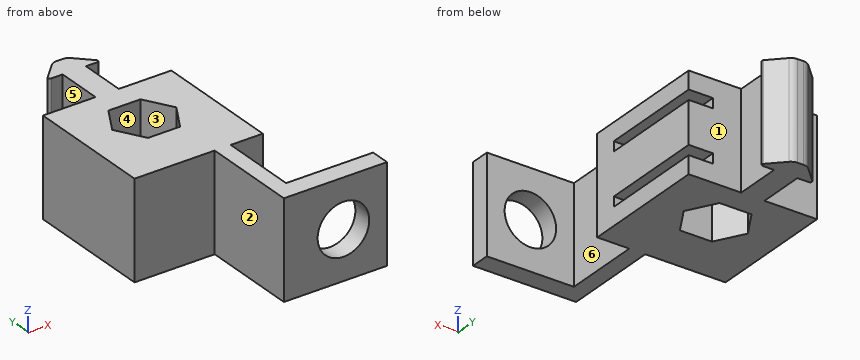
```python
from build123d import *

# Parameters (mm, degrees)
BOSS_EXTRUDE1_DEPTH = 12.7
SKETCH8_W           = 2.54
SKETCH8_H           = 27.5
CUT_EXTRUDE1_DEPTH  = 6.35
SKETCH3_W           = 4.197769469
SKETCH3_H           = 25.4
BOSS_EXTRUDE2_DEPTH = 25.4
SKETCH4_W           = 22.800422122
SKETCH4_H           = 25.4
SKETCH4_R           = 6.75
BOSS_EXTRUDE3_DEPTH = 5.08


with BuildPart() as part:
    # Sketch1 → Boss-Extrude1 (new body, symmetric)
    with BuildSketch(Plane.XY):
        with BuildLine():
            Line((-16.79575, 13.62075), (-16.79575, -19.97075))
            Line((-16.79575, -19.97075), (16.79575, -19.97075))
            Line((16.79575, -19.97075), (16.79575, 13.62075))
            Line((16.79575, 13.62075), (3.048, 13.62075))
            Line((3.048, 13.62075), (3.048, 25.68575))
            Line((3.048, 25.68575), (6.01257951, 25.68575))
            ThreePointArc((6.01257951, 25.68575), (6.481910313, 25.999346816), (6.371789755, 26.552960245))
            Line((6.371789755, 26.552960245), (2.532108776, 30.392641224))
            ThreePointArc((2.532108776, 30.392641224), (1.70807347, 30.943244013), (0.736057552, 31.13659))
            Line((0.736057552, 31.13659), (-0.736057552, 31.13659))
            ThreePointArc((-0.736057552, 31.13659), (-1.70807347, 30.943244013), (-2.532108776, 30.392641224))
            Line((-2.532108776, 30.392641224), (-6.371789755, 26.552960245))
            ThreePointArc((-6.371789755, 26.552960245), (-6.481910313, 25.999346816), (-6.01257951, 25.68575))
            Line((-6.01257951, 25.68575), (-3.048, 25.68575))
            Line((-3.048, 25.68575), (-3.048, 13.62075))
            Line((-3.048, 13.62075), (-16.79575, 13.62075))
        make_face()
        Polygon((-4.19776947, 7.27075), (-8.395538939, 0), (-4.19776947, -7.27075), (4.19776947, -7.27075), (8.395538939, 0), (4.19776947, 7.27075), align=None, mode=Mode.SUBTRACT)
    extrude(amount=BOSS_EXTRUDE1_DEPTH, both=True)

    # Sketch8 → Cut-Extrude1 (cut)
    with BuildSketch(Plane(origin=(16.79575, 0, 0), x_dir=(0, 0, -1), z_dir=(1, 0, 0))):
        with Locations((-6.77, -0.12925)):
            Rectangle(SKETCH8_W, SKETCH8_H)
        with Locations((6.77, -0.12925)):
            Rectangle(SKETCH8_W, SKETCH8_H)
    extrude(amount=-CUT_EXTRUDE1_DEPTH, mode=Mode.SUBTRACT)

    # Sketch3 → Boss-Extrude2 (add)
    with BuildSketch(Plane.XZ.offset(19.97075)):
        with Locations((6.296654204, 0)):
            Rectangle(SKETCH3_W, SKETCH3_H)
    extrude(amount=BOSS_EXTRUDE2_DEPTH)

    # Sketch4 → Boss-Extrude3 (add)
    with BuildSketch(Plane.XZ.offset(45.37075)):
        with Locations((19.79575, 0)):
            Rectangle(SKETCH4_W, SKETCH4_H)
        with Locations((19.79575, 0)):
            Circle(SKETCH4_R, mode=Mode.SUBTRACT)
    extrude(amount=-BOSS_EXTRUDE3_DEPTH)


solid = part.part
```
For this review, take the finished solid that the model builds, in its own axes (mm). Face numbers are marked on the shaded views. A direction names the side the tool comes from. Coordinates: 2 decimals unless noted, no trailing zeros. Write each loop counter-clockwise with the first axis right and the second up, starting at its lowest first coordinate (ties: lowest second). Pieces come first, ordered by that corner, then holes.
(1) For pin 1 Ø6 at (y, z) = (-34.5, 7) entering from -X; pin 2 Ø1.5 at (x, z) = (5.5, -6) entering from +Y; pin 3 Ø0.9 at (x, z) = (-5, -6) entering from -Y, all flat-tipped, find the tip position at first contact; note any pin that passes through.
(2) Add section C-C on y = 8.5. Give the boundary of the cut face in (x, z), then the cut area to 3 significant figures.
(3) Tool access review of the marked faces 4, 5 and 6: name each direction out of +Z, -Z, +X, -X, +Y, -Y from which nothing blocks a thin tool from reaching the whole face with its end or side.
(4) Add section A-A on z = 0. Count the separate pieces of the cut face and the enclosed holes in it, then the cut area to 3 significant figures.
(5) Add section B-B on z = -9.5. Give the boundary of the cut face in (x, y).
(6) The part is to be moulded in two halves that separate along X. For the marked faces 1, 2 and 3, say which applies: +X half, -X half, draft (parallel to the pull), parting line (faces both ways), or undercut.
(7) Wall thickness on probe 1 along Y at (x, z) = (12, 7.5); probe 2 along Y at (x, z) = (11, -3); probe 3 along X at (y, z) = (-5, 4.75): over which ranges is each line inside the solid? List them lowest first.
Answer sheet:
1. pin 1: stops at x = 4.2
1. pin 2: stops at y = 28.17
1. pin 3: stops at y = -19.97
2. outline: (-16.8, -12.7) - (16.8, -12.7) - (16.8, -8.04) - (10.45, -8.04) - (10.45, -5.5) - (16.8, -5.5) - (16.8, 5.5) - (10.45, 5.5) - (10.45, 8.04) - (16.8, 8.04) - (16.8, 12.7) - (-16.8, 12.7) - close
2. area: 821 mm2
3. face 4: +Z, -Z
3. face 5: +Z, -Z, -X
3. face 6: +Z, -Z, +X
4. separate pieces: 2
4. enclosed holes: 1
4. area: 1,220 mm2
5. outline: (-16.8, -19.97) - (4.2, -19.97) - (4.2, -45.37) - (31.2, -45.37) - (31.2, -40.29) - (8.4, -40.29) - (8.4, -19.97) - (16.8, -19.97) - (16.8, 13.62) - (3.05, 13.62) - (3.05, 25.69) - (6.01, 25.69) arc R0.51 ccw to (6.37, 26.55) - (2.53, 30.39) arc R2.54 ccw to (0.74, 31.14) - (-0.74, 31.14) arc R2.54 ccw to (-2.53, 30.39) - (-6.37, 26.55) arc R0.51 ccw to (-6.01, 25.69) - (-3.05, 25.69) - (-3.05, 13.62) - (-16.8, 13.62) - close; hole (-8.4, 0) - (-4.2, -7.27) - (4.2, -7.27) - (8.4, 0) - (4.2, 7.27) - (-4.2, 7.27) - close
6. face 1: draft
6. face 2: -X half
6. face 3: undercut
7. probe 1: y = -45.37 to -40.29, -19.97 to -13.88
7. probe 2: y = -45.37 to -40.29, -19.97 to 13.62
7. probe 3: x = -16.8 to -5.51, 5.51 to 16.8
